Could you check a few things on this model? Use its own coordinates, in mm. Face numbers are marked on the shaded views. Coordinates: 2 decimals unless noted, no trailing zeros. Order: outer loops, then holes, each group sorted by start corner. A loop starts at its lowest first (then second) coordinate and runs counter-clockwise, first axis right, second up. Notation, with made-up numbers: M 32,87 L 82,87 A13 ccw 82,97 Z; hole C 22,41 d11. An arc over 180 degrees is marked long. One line per question, with ' | ' between items. Start each with the question number.
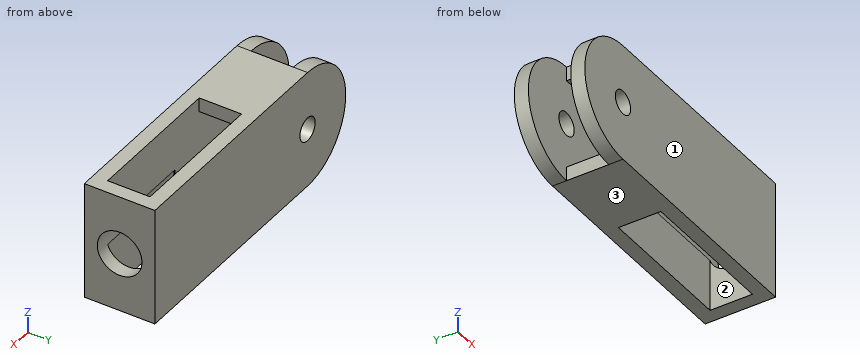
from build123d import *

# Parameters (mm, degrees)
SKETCH1_R               = 5
BOSS_EXTRUDE1_DEPTH     = 15
SKETCH5_R               = 9.5
CUT_EXTRUDE1_DEPTH      = 50
CUT_EXTRUDE2_DEPTH      = 81.467384697
CUT_EXTRUDE2_DEPTH_BACK = 81.467384697
SKETCH6_W               = 60
SKETCH6_H               = 18
SKETCH6_W_2             = 25
SKETCH7_W               = 38
SKETCH7_H               = 18
CUT_EXTRUDE3_DEPTH      = 73.15261603


with BuildPart() as part:
    # Sketch1 → Boss-Extrude1 (new, symmetric)
    with BuildSketch(Plane(origin=(0, 0, 0), x_dir=(1, 0, 0), z_dir=(0, 1, 0))):
        with BuildLine():
            Line((-50, 25), (50, 25))
            Line((50, 25), (50, -25))
            Line((50, -25), (-50, -25))
            ThreePointArc((-50, -25), (-75, 0), (-50, 25))
        make_face()
        with Locations(Location((-50, 0, 0), (0, 0, 270))):
            Circle(SKETCH1_R, mode=Mode.SUBTRACT)
    extrude(amount=BOSS_EXTRUDE1_DEPTH, both=True)

    # Sketch5 → Cut-Extrude1 (cut)
    with BuildSketch(Plane(origin=(50, 0, 0), x_dir=(0, 0, -1), z_dir=(1, 0, 0))):
        Circle(SKETCH5_R)
    extrude(amount=-CUT_EXTRUDE1_DEPTH, mode=Mode.SUBTRACT)

    # Sketch6 → Cut-Extrude2 (cut, two sides: drawn at the far end of the back side and taken through both)
    with BuildSketch(Plane.XY.offset(-CUT_EXTRUDE2_DEPTH_BACK)):
        with Locations((14, 0)):
            Rectangle(SKETCH6_W, SKETCH6_H)
        with Locations((-62.5, 0)):
            Rectangle(SKETCH6_W_2, SKETCH6_H)
    extrude(amount=CUT_EXTRUDE2_DEPTH + CUT_EXTRUDE2_DEPTH_BACK, mode=Mode.SUBTRACT)

    # Sketch7 → Cut-Extrude3 (cut, through all)
    with BuildSketch(Plane(origin=(-16, 0, 0), x_dir=(0, 0, -1), z_dir=(1, 0, 0))):
        Rectangle(SKETCH7_W, SKETCH7_H)
    extrude(amount=-CUT_EXTRUDE3_DEPTH, mode=Mode.SUBTRACT)


solid = part.part
(1) We'd pull the mould along Y, two halves only. Please class the marked faces 1, 2 and 3: +Y half, -Y half, draft (parallel to the pull), parting line (faces both ways), or undercut.
(2) Imagine slicing it at A-A, the plane z = 0. Write out the boundary of the cut face in (x, y), plus the area to 3 significant figures.
(3) Imagine slicing it at D-D, the plane x = -37. Write out the boundary of the cut face in (y, z).
(4) For P1, Ø9, axis at y = 2, z = 12, coming from the -X side; P2, Ø12, axis at y = 4, z = -0.5, coming from the -X side; P3, Ø6.5, axis at y = 1, z = 22.5, coming from the -X side; P4, Ø10, axis at x = 12.5, y = -1, coming from the -Z side (3 decimals), each with a flat end and sliding along its axis, tell me the tip position at first contact or that it passes through.
(5) If I drill on line 1 along X through (y, z) = (4, -20); line 2 along Y through (x, z) = (15.5, 14); line 3 along Y through (x, z) = (39, 0), over which ranges is the centre line in solid material (lowest first)? Write a range as from..to.
(6) Imagine slicing it at C-C, the plane y = 0. Write out the boundary of the cut face in (x, z), plus the area to 3 significant figures.
(7) Imagine slicing it at B-B, the plane x = 17.5. Write out the boundary of the cut face in (y, z), plus the area to 3 significant figures.
Answers:
1) face 1: -Y half | face 2: undercut | face 3: draft
2) outline: M -75,-15 L -55,-15 L -55,-9 L -75,-9 Z; M -75,9 L -55,9 L -55,15 L -75,15 Z; M -45,-15 L 50,-15 L 50,-9.5 L 0,-9.5 L 0,-9 L -45,-9 Z; M -45,9 L 0,9 L 0,9.5 L 50,9.5 L 50,15 L -45,15 Z | area: 1,330 mm²
3) outline: M -15,-25 L 15,-25 L 15,25 L -15,25 Z; hole M -9,-19 L 9,-19 L 9,19 L -9,19 Z
4) P1: x = 44 | P2: x = -75 | P3: x = -50 | P4: through
5) line 1: -50..-16, 44..50 | line 2: -15..-9, 9..15 | line 3: -15..-9.5, 9.5..15
6) outline: M -50,-25 L -16,-25 L -16,-19 L -50,-19 Z; M -50,19 L -16,19 L -16,25 L -50,25 Z; M 44,-25 L 50,-25 L 50,-9.5 L 44,-9.5 Z; M 44,9.5 L 50,9.5 L 50,25 L 44,25 Z | area: 594 mm²
7) outline: M -15,-25 L -9,-25 L -9,-3.04 A9.5 cw -9,3.04 L -9,25 L -15,25 Z; M 9,-25 L 15,-25 L 15,25 L 9,25 L 9,3.04 A9.5 cw 9,-3.04 Z | area: 596 mm²
